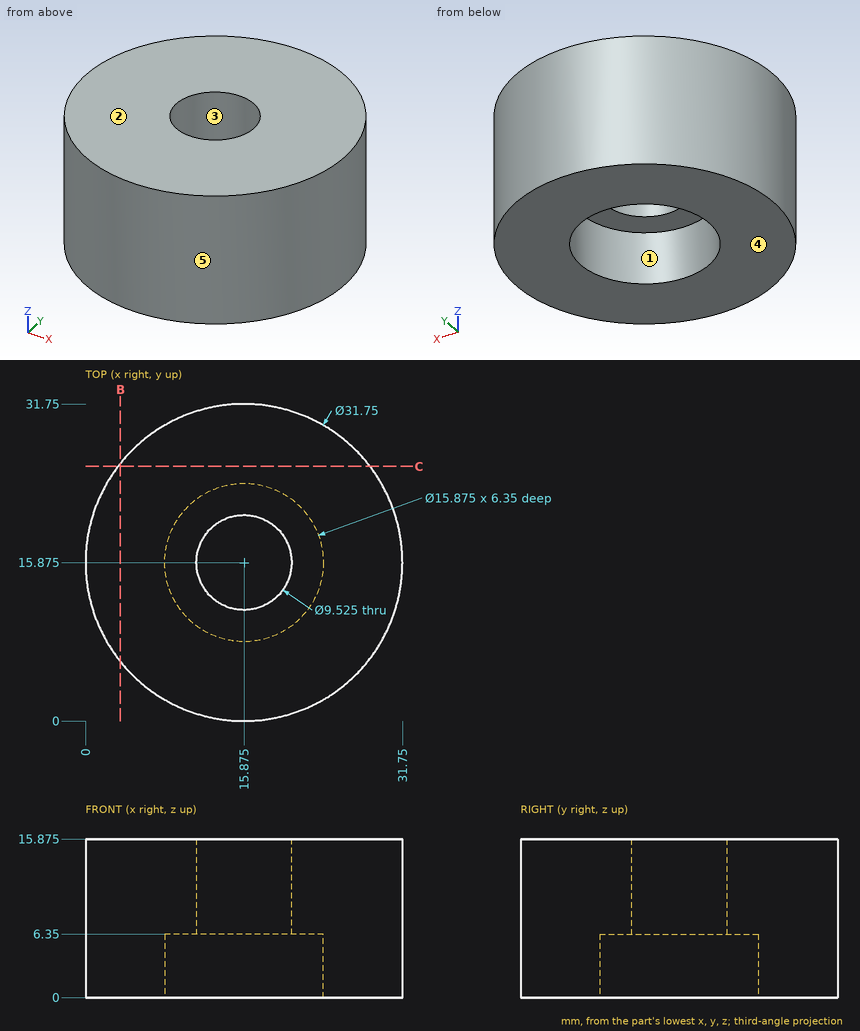
Input: dimensioned drawing with shaded views. Units: mm. Origin: part minimum x, y, z. A direction names the side the tool comes from. Give positions to 0.01 mm unless a question says otherwise; leave off trailing zeros. Loops run counter-clockwise (first coordinate to the right, second up) from the corner with the lowest first, then second, coordinate; pieces in that order, holes last. Notation, with made-up numbers: M 40.25,72 L 71.25,72 A31 cw 71.25,98 Z; hole C 55.5,63.5 d1. An arc over 180 degrees is marked long. Put each result on its own line as item: value.
1) Reachability of the marked faces 1 and 2 from +Z, -Z, +X, -X, +Y, -Y: full face, straight path, thin tool, end or side. Return the list, or none.
Computed values:
face 1: -Z
face 2: +Z, +X, -X, +Y, -Y
2) Cut plane B-B, the plane x = 3.5. Return the cut outline in (y, z) (3 decimals).
Computed values:
outline: M 5.931,0 L 25.819,0 L 25.819,15.875 L 5.931,15.875 Z
3) Mould query, pull axis X, two halves, no side actions, for the marked faces 3, 4 and 5. Classes: released by +X, released by -X, zero draft, split by the parting line, or undercut.
Computed values:
face 3: undercut
face 4: zero draft
face 5: split by the parting line
4) Cut plane C-C, the plane y = 25.5. Return the cut outline in (x, z) (3 decimals).
Computed values:
outline: M 3.251,0 L 28.499,0 L 28.499,15.875 L 3.251,15.875 Z
5) Material intervals for L1, parallel to X at y = 16, z = 3; L2, parallel to Y at x = 15.5, z = 1.5; L3, parallel to X at y = 13, z = 2.25, sorted ascending. Write a range as from..to.
Computed values:
L1: x = 0..7.94, 23.81..31.75
L2: y = 0..7.95, 23.8..31.75
L3: x = 0.26..8.48, 23.27..31.49
6) First-contact query: P1, Ø3, axis at y = 24.5, z = 7, coming from the -X side; P2, Ø1.5, axis at y = 28, z = 7.5, coming from the -X side; P3, Ø8, axis at x = 21.5, z = 10.5, coming from the -Y side. Flat tips, straight axial feed; report the tip coordinate or a pass-through.
Computed values:
P1: stops at x = 1.69
P2: stops at x = 4.8
P3: stops at y = 0.08
